Check sheet for the modelled part. Datum: model origin and axes. Units: mm. Coordinates: 2 decimals unless noted, no trailing zeros. Write each loop counter-clockwise with the first axis right and the second up, starting at its lowest first coordinate (ties: lowest second). Pieces come first, ordered by that corner, then holes. Notation, with made-up numbers: (20, 22.25) -> (51, 22.25) arc R17 cw to (51, 37.25) -> close; hole circle Ø2 at (85.5, 16.25). An arc over 180 degrees is marked (long way). Put each result on its own line as item: value.
```python
from build123d import *

# Parameters (mm, degrees)
EXTRUDE_1_DEPTH     = 8
SKETCH_2_R          = 11
SKETCH_2_R_2        = 5.75
EXTRUDE_2_DEPTH     = 27
CUT_EXTRUDE_START   = -27
SKETCH_3_R          = 5.75
CUT_EXTRUDE_1_DEPTH = 27
SKETCH_4_R          = 43.168143545
SKETCH_4_R_2        = 20
CUT_EXTRUDE_2_DEPTH = 27
SKETCH_5_R          = 1.5
CUT_EXTRUDE_3_DEPTH = 40.102429592
CHAMFER_1_SIZE      = 0.5


with BuildPart() as part:
    # 草图1 → 凸台-拉伸1 (new body)
    with BuildSketch(Plane(origin=(0, 0, 0), x_dir=(1, 0, 0), z_dir=(0, 1, 0))):
        with BuildLine():
            Line((6.085610762, 25.384237528), (-25.942357498, -2.896249422))
            ThreePointArc((-25.942357498, -2.896249422), (-19.567194229, -17.277704803), (-6.085610762, -25.384237528))
            Line((-6.085610762, -25.384237528), (25.942357498, 2.896249422))
            ThreePointArc((25.942357498, 2.896249422), (19.567194229, 17.277704803), (6.085610762, 25.384237528))
        make_face()
    extrude(amount=EXTRUDE_1_DEPTH)

    # 草图2 → 凸台-拉伸2 (add)
    with BuildSketch(Plane(origin=(0, 8, 0), x_dir=(1, 0, 0), z_dir=(0, 1, 0))):
        with Locations(Location((0, 0, 0), (0, 0, 270))):
            Circle(SKETCH_2_R)
        with Locations(Location((0, 0, 0), (0, 0, 270))):
            Circle(SKETCH_2_R_2, mode=Mode.SUBTRACT)
    extrude(amount=EXTRUDE_2_DEPTH)

    # 草图3 → 切除-拉伸1 (cut)
    with BuildSketch(Plane(origin=(0, 8, 0), x_dir=(1, 0, 0), z_dir=(0, 1, 0)).offset(CUT_EXTRUDE_START)):
        with Locations(Location((0, 0, 0), (0, 0, 270))):
            Circle(SKETCH_3_R)
    extrude(amount=CUT_EXTRUDE_1_DEPTH, mode=Mode.SUBTRACT)

    # 草图4 → 切除-拉伸2 (cut)
    with BuildSketch(Plane(origin=(0, 8, 0), x_dir=(1, 0, 0), z_dir=(0, 1, 0))):
        Circle(SKETCH_4_R)
        Circle(SKETCH_4_R_2, mode=Mode.SUBTRACT)
    extrude(amount=-CUT_EXTRUDE_2_DEPTH, mode=Mode.SUBTRACT)

    # 草图5 → 切除-拉伸3 (cut, through all)
    with BuildSketch(Plane(origin=(0, 8, 0), x_dir=(1, 0, 0), z_dir=(0, 1, 0))):
        with Locations(Location((0.983422311, 15.96974892, 0), (0, 0, 270))):
            Circle(SKETCH_5_R)
        with Locations(Location((11.98770234, 10.59693317, 0), (0, 0, 270))):
            Circle(SKETCH_5_R)
        with Locations(Location((15.96974892, -0.983422311, 0), (0, 0, 270))):
            Circle(SKETCH_5_R)
        with Locations(Location((-0.983422311, -15.96974892, 0), (0, 0, 270))):
            Circle(SKETCH_5_R)
        with Locations(Location((-11.98770234, -10.59693317, 0), (0, 0, 270))):
            Circle(SKETCH_5_R)
        with Locations(Location((-15.96974892, 0.983422311, 0), (0, 0, 270))):
            Circle(SKETCH_5_R)
    extrude(amount=-CUT_EXTRUDE_3_DEPTH, mode=Mode.SUBTRACT)

    # 倒角1
    chamfer_1_edges = [part.edges().sort_by_distance(p)[0] for p in [
        (0, 35, -11),
        (0, 8, -11),
        (0, 35, -5.75),
        (0, 0, -5.75),
        (9.928373368, 0, 11.243994053),
        (-9.928373368, 0, -11.243994053),
        (-14.991992071, 0, 13.237831157),
        (14.991992071, 0, -13.237831157),
        (9.928373368, 8, 11.243994053),
        (-9.928373368, 8, -11.243994053),
        (14.991992071, 8, -13.237831157),
        (-14.991992071, 8, 13.237831157),
        (0.983422311, 0, -17.46974892),
        (0.983422311, 8, -17.46974892),
        (11.98770234, 0, -12.09693317),
        (11.98770234, 8, -12.09693317),
        (15.96974892, 0, -0.516577689),
        (15.96974892, 8, -0.516577689),
        (-0.983422311, 0, 14.46974892),
        (-0.983422311, 8, 14.46974892),
        (-11.98770234, 0, 9.09693317),
        (-11.98770234, 8, 9.09693317),
        (-15.96974892, 0, -2.483422311),
        (-15.96974892, 8, -2.483422311),
    ]]
    chamfer(chamfer_1_edges, length=CHAMFER_1_SIZE)


solid = part.part
```
Q1. Depth check by flat-ended pin: P1, Ø1.8, axis at x = -15.97, z = -0.98, coming from the -Y side; P2, Ø4, axis at y = 23, z = -2.5, coming from the +X side; P3, Ø3.5, axis at x = -11.99, z = 10.6, coming from the -Y side; P4, Ø2, axis at x = 4, y = 24.5, coming from the -Z side. Enter the tip coordinate at first touch or a pass-through.
Recorded:
P1: passes through
P2: stops at x = 10.99
P3: stops at y = 0.25
P4: stops at z = -10.58
Q2. Mould release check, pull along X, two halves, no side actions. Record for faces 1 (the flat face through (-9.79, 3.951, -11.367)), 2 (the cylindrical face through (-10.74, 21.32, -2.38)), 3 (the cylindrical face through (1.05, 4.05, -17.47)): released by +X, released by -X, zero draft, split by the parting line, or undercut.
Recorded:
face 1: released by -X
face 2: split by the parting line
face 3: undercut
Q3. Material ranges on line 1 along X through (y, z) = (28.5, 0); line 2 along Y through (x, z) = (7, -10.5); line 3 along Z through (x, y) = (4, 33.5), recorded low to high.
Recorded:
line 1: x = -11 to -5.75, 5.75 to 11
line 2: y = 0 to 8
line 3: z = -10.25 to -4.13, 4.13 to 10.25
Q4. Cross-section at A-A (y = 11). Record the cut outline in (x, z), plus the area to 3 significant figures.
Recorded:
outline: circle Ø22 at (0, 0); hole circle Ø11.5 at (0, 0)
area: 276 mm2
